Verification items for this drawing (mm, ordinates from the low corner). Coordinates: 2 decimals unless noted, no trailing zeros. Loops run counter-clockwise (first coordinate to the right, second up) from the corner with the lowest first, then second, coordinate; pieces in that order, holes last. Notation, with made-up numbers: M -30,-7 L -10,-7 A23 ccw -10,28 Z; hole C 4.25,68 d1. An arc over 180 degrees is marked long. Use CSV: the item, a comma, the result in double quotes.
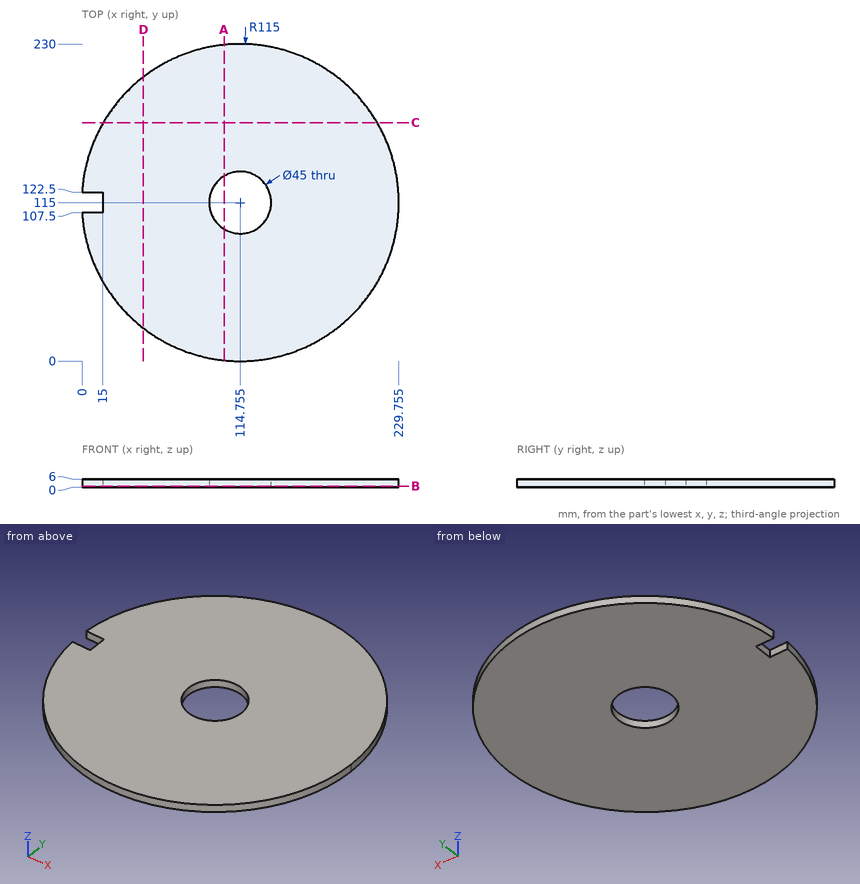
1. Section check D-D, the plane x = 44.5. Record the cut outline in (y, z) (3 decimals).
The answers:
outline,"M 23.955,0 L 206.045,0 L 206.045,6 L 23.955,6 Z"
2. Section check A-A, the plane x = 103. Record the cut outline in (y, z) (1 decimal).
The answers:
outline,"M 0.6,0 L 95.8,0 L 95.8,6 L 0.6,6 Z; M 134.2,0 L 229.4,0 L 229.4,6 L 134.2,6 Z"
3. Thickness scan on line 1 (X direction, y = 121.5, z = 5.1) (1 decimal); line 2 (Y direction, x = 63.5, z = 5.85); line 3 (X direction, y = 46.5, z = 3.8). Record the ranges inside material, lowest first. Write a range as [from, to].
The answers:
line 1,"[15, 93.2], [136.3, 229.6]"
line 2,"[12.05, 217.95]"
line 3,"[22.38, 207.13]"
4. Section check B-B, the plane z = 0.9. Record the cut outline in (x, y) (1 decimal).
The answers:
outline,"M 0,107.5 A115 ccw long 0,122.5 L 15,122.5 L 15,107.5 Z; hole C 114.8,115 d45"
5. Gauge pin test, flat ends, axial feed: P1, Ø2, axis at y = 84.5, z = 5, coming from the +X side; P2, Ø2, axis at x = 114, z = 4, coming from the +Y side; P3, Ø1.8, axis at x = 9, z = 4, coming from the +Y side. Record the tip position at first contact, or that the pin passes through.
The answers:
P1,"x = 225.91"
P2,"y = 230"
P3,"y = 162.23"
6. Section check C-C, the plane y = 173. Record the cut outline in (x, z), plus the area to 3 significant figures.
The answers:
outline,"M 15.45,0 L 214.06,0 L 214.06,6 L 15.45,6 Z"
area,"1,190 mm^2"
